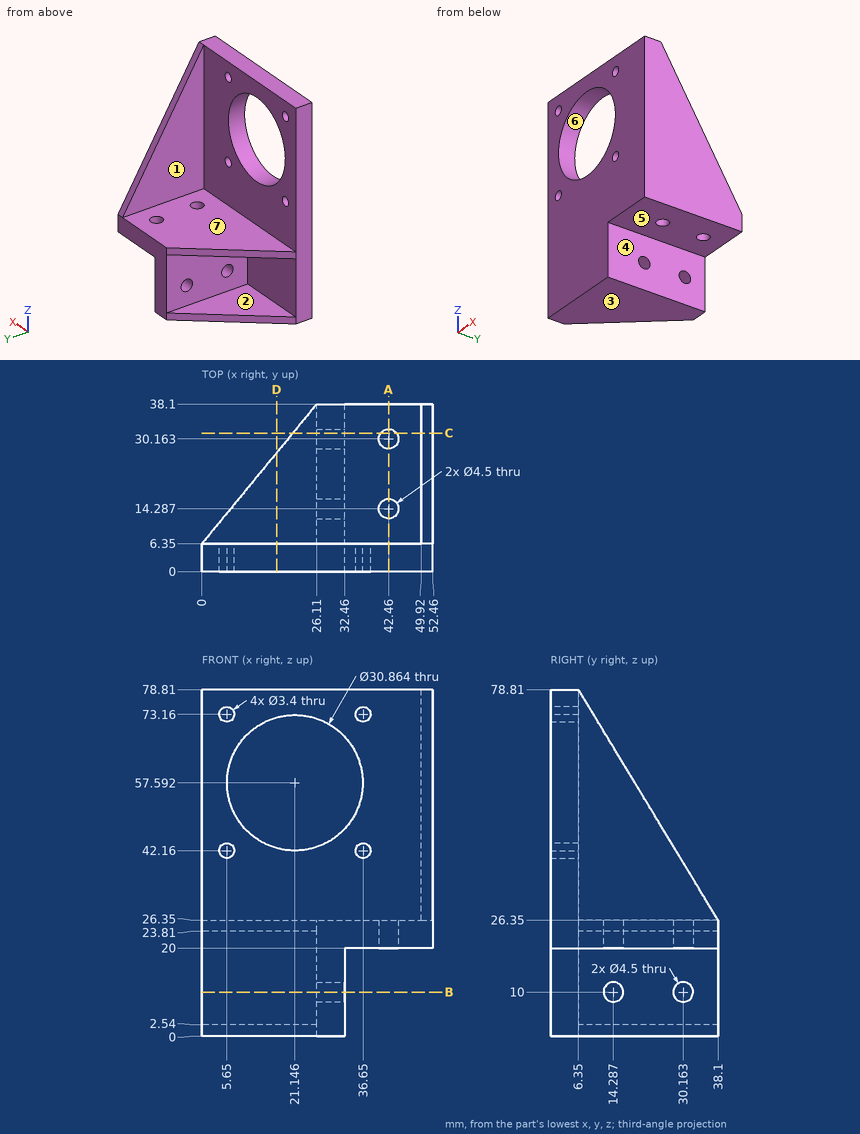
Job drawing, mm, ordinate dimensions from the low corner. One solid piece. A direction names the side the tool comes from. Coordinates: 2 decimals unless noted, no trailing zeros. Order: outer loops, then holes, each group sorted by start corner. A loop starts at its lowest first (then second) coordinate and runs counter-clockwise, first axis right, second up. Notation, with made-up numbers: (72, 75) -> (82, 75) arc R19 cw to (82, 87) -> close; hole circle Ø9 at (45, 35). An arc over 180 degrees is marked (long way). Answer in a Markdown table with one row per item. Add a question column.
Q1. Band-saw the part on A-A, the plane x = 42.46. List the corners of the cut face in (y, z), then the cut area to 3 significant figures.
Q2. Band-saw the part on B-B, the plane z = 10. List the corners of the cut face in (x, y).
Q3. Band-saw the part on C-C, the plane y = 31.5. Give the number of separate pieces and of enclosed holes in the cut face.
Q4. Mould opens along Z. For the marked faces 4, 5, 6 and 7 say: +Z half, -Z half, draft (parallel to the pull), parting line (faces both ways), or undercut.
Q5. Wall check: line 1 along Y through (x, z) = (29.75, 10); line 2 along Z through (x, y) = (20, 26.5); line 3 along Z through (x, y) = (46, 3). Give the ranges that are in metal, low to high. Write a range as [from, to].
Q6. Band-saw the part on D-D, the plane x = 17. List the corners of the cut face in (y, z).
Q7. Which spindle directions (+Z, -Z, +X, -X, +Y, -Y) get a long thin tool onto all of the face, cutting with end or side? Do the marked faces 1, 2 and 3. Say none if no direction does.
Q8. Drop flat-ended pins along their axis: pin 1 (21 mm diameter, centred on x = 14.5, y = 21.5, fed in from +Z); pin 2 (16 mm diameter, centred on y = 20, z = 9, fed in from +X); pin 3 (3 mm diameter, centred on x = 42.5, y = 4, fed in from -Z). Give the stop position or say it passes through.
Answers follow:
| question | item | result |
|---|---|---|
| 1 | outline | (0, 20) -> (12.04, 20) -> (12.04, 26.35) -> (6.35, 26.35) -> (6.35, 78.81) -> (0, 78.81) -> close; (16.54, 20) -> (27.91, 20) -> (27.91, 26.35) -> (16.54, 26.35) -> close; (32.41, 20) -> (38.1, 20) -> (38.1, 26.35) -> (32.41, 26.35) -> close |
| 1 | area | 518 mm^2 |
| 2 | outline | (0, 0) -> (32.46, 0) -> (32.46, 12.04) -> (26.11, 12.04) -> (26.11, 6.35) -> (0, 6.35) -> close; (26.11, 16.54) -> (32.46, 16.54) -> (32.46, 27.91) -> (26.11, 27.91) -> close; (26.11, 32.41) -> (32.46, 32.41) -> (32.46, 38.1) -> (26.11, 38.1) -> close |
| 3 | separate pieces | 3 |
| 3 | enclosed holes | 0 |
| 4 | face 4 | draft |
| 4 | face 5 | -Z half |
| 4 | face 6 | undercut |
| 4 | face 7 | +Z half |
| 5 | line 1 | [0, 12.04], [16.54, 27.91], [32.41, 38.1] |
| 5 | line 2 | [0, 2.54], [23.81, 26.35] |
| 5 | line 3 | [20, 78.81] |
| 6 | outline | (0, 0) -> (27.02, 0) -> (27.02, 2.54) -> (6.35, 2.54) -> (6.35, 23.81) -> (27.02, 23.81) -> (27.02, 26.35) -> (6.35, 26.35) -> (6.35, 42.73) -> (0, 42.73) -> close; (0, 72.46) -> (6.35, 72.46) -> (6.35, 78.81) -> (0, 78.81) -> close |
| 7 | face 1 | +Z, -X, +Y |
| 7 | face 2 | -X, +Y |
| 7 | face 3 | -Z, +X, -X, +Y, -Y |
| 8 | pin 1 | z = 26.35 |
| 8 | pin 2 | x = 32.46 |
| 8 | pin 3 | z = 20 |
